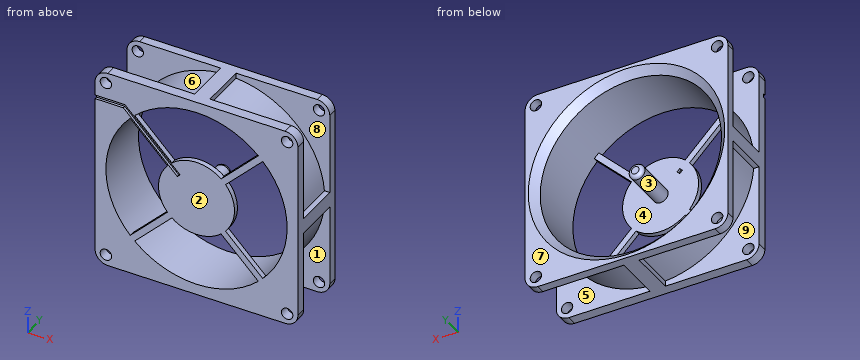
```python
from build123d import *

# Parameters (mm, degrees)
SKETCH1_W            = 80
SKETCH1_H            = 80
BOSS_EXTRUDE1_DEPTH  = 25.5
SKETCH2_R            = 35.75
CUT_EXTRUDE2_DEPTH   = 28
BOSS_EXTRUDE2_DEPTH  = 2
CIRPATTERN2_COUNT    = 4
SKETCH5_R            = 15
BOSS_EXTRUDE3_DEPTH  = 2
SKETCH6_R            = 3
BOSS_EXTRUDE4_DEPTH  = 17.5
FILLET1_R            = 1.5
SKETCH7_R            = 70
SKETCH7_R_2          = 38
CUT_EXTRUDE4_DEPTH   = 18
FILLET2_R            = 5
BOSS_EXTRUDE5_DEPTH  = 20
CIRPATTERN3_COUNT    = 4
SKETCH9_R            = 2.25
CUT_EXTRUDE5_DEPTH   = 37
LPATTERN1_COUNT      = 2
LPATTERN1_PITCH      = 71.5
LPATTERN1_COUNT_DIR2 = 2
LPATTERN1_PITCH_DIR2 = 71.5
CHAMFER2_SIZE        = 3
CUT_EXTRUDE6_DEPTH   = 1
CUT_EXTRUDE7_DEPTH   = 7


with BuildPart() as part:
    # Sketch1 → Boss-Extrude1 (new body)
    with BuildSketch(Plane(origin=(0, 0, 0), x_dir=(1, 0, 0), z_dir=(0, 1, 0))):
        Rectangle(SKETCH1_W, SKETCH1_H)
    extrude(amount=BOSS_EXTRUDE1_DEPTH)

    # Sketch2 → Cut-Extrude2 (cut)
    with BuildSketch(Plane(origin=(0, 25.5, 0), x_dir=(1, 0, 0), z_dir=(0, 1, 0))):
        Circle(SKETCH2_R)
    extrude(amount=-CUT_EXTRUDE2_DEPTH, mode=Mode.SUBTRACT)

    # Sketch4 → Boss-Extrude2 (add)
    with BuildSketch(Plane.XZ):
        with BuildLine():
            Line((-1.75, 0), (0, 1.785533906))
            Line((0, 1.785533906), (-24.370530875, 26.156064781))
            ThreePointArc((-24.370530875, 26.156064781), (-25.270176953, 25.287954776), (-26.138919431, 24.388919431))
            Line((-26.138919431, 24.388919431), (-1.75, 0))
        make_face()
    boss_extrude2 = extrude(amount=-BOSS_EXTRUDE2_DEPTH)

    # CirPattern2: Boss-Extrude2 ×4 about axis
    cirpattern2_axis = Axis((0, 0, 0), (0, 1, 0))
    for i in range(1, CIRPATTERN2_COUNT):
        add(boss_extrude2.rotate(cirpattern2_axis, i * 360 / CIRPATTERN2_COUNT))

    # Sketch5 → Boss-Extrude3 (add)
    with BuildSketch(Plane.XZ):
        Circle(SKETCH5_R)
    extrude(amount=-BOSS_EXTRUDE3_DEPTH)

    # Sketch6 → Boss-Extrude4 (add)
    with BuildSketch(Plane(origin=(0, 2, 0), x_dir=(1, 0, 0), z_dir=(0, 1, 0))):
        Circle(SKETCH6_R)
    extrude(amount=BOSS_EXTRUDE4_DEPTH)

    # Fillet1
    fillet1_edges = [part.edges().sort_by_distance(p)[0] for p in [
        (-3, 19.5, 0),
    ]]
    fillet(fillet1_edges, radius=FILLET1_R)

    # Sketch7 → Cut-Extrude4 (cut)
    with BuildSketch(Plane.XZ.offset(-4)):
        Circle(SKETCH7_R)
        Circle(SKETCH7_R_2, mode=Mode.SUBTRACT)
    extrude(amount=-CUT_EXTRUDE4_DEPTH, mode=Mode.SUBTRACT)

    # Fillet2
    fillet2_edges = [part.edges().sort_by_distance(p)[0] for p in [
        (-40, 2, -40),
        (40, 2, -40),
        (40, 2, 40),
        (-40, 2, 40),
        (-40, 23.75, -40),
        (40, 23.75, -40),
        (40, 23.75, 40),
        (-40, 23.75, 40),
    ]]
    fillet(fillet2_edges, radius=FILLET2_R)

    # Sketch8 → Boss-Extrude5 (add)
    with BuildSketch(Plane.XZ.offset(-4)):
        with BuildLine():
            Line((-3, 40), (3, 40))
            Line((3, 40), (3, 35.623903492))
            ThreePointArc((3, 35.623903492), (0, 35.75), (-3, 35.623903492))
            Line((-3, 35.623903492), (-3, 40))
        make_face()
    boss_extrude5 = extrude(amount=-BOSS_EXTRUDE5_DEPTH)

    # CirPattern3: Boss-Extrude5 ×4 about axis
    cirpattern3_axis = Axis((0, 0, 0), (0, 1, 0))
    for i in range(1, CIRPATTERN3_COUNT):
        add(boss_extrude5.rotate(cirpattern3_axis, i * 360 / CIRPATTERN3_COUNT))

    # Sketch9 → Cut-Extrude5 (cut)
    with BuildSketch(Plane(origin=(0, 25.5, 0), x_dir=(-1, 0, 0), z_dir=(0, 1, 0))):
        with Locations((35.75, -35.75)):
            Circle(SKETCH9_R)
    cut_extrude5 = extrude(amount=-CUT_EXTRUDE5_DEPTH, mode=Mode.SUBTRACT)

    # LPattern1: Cut-Extrude5 2 × 2
    with Locations(*[(i * LPATTERN1_PITCH, 0, j * LPATTERN1_PITCH_DIR2) for i in range(LPATTERN1_COUNT) for j in range(LPATTERN1_COUNT_DIR2) if (i, j) != (0, 0)]):
        add(cut_extrude5, mode=Mode.SUBTRACT)

    # Chamfer2
    chamfer2_edges = [part.edges().sort_by_distance(p)[0] for p in [
        (-35.75, 25.5, 0),
    ]]
    chamfer(chamfer2_edges, length=CHAMFER2_SIZE)

    # Sketch11 → Cut-Extrude6 (cut)
    with BuildSketch(Plane.XZ):
        Polygon((-28.863216429, 27.820323211), (-7.554875149, 6.51198193), (-6.494214977, 7.572642102), (-28.241896086, 29.320323211), (-40, 29.320323211), (-40, 27.820323211), align=None)
    extrude(amount=-CUT_EXTRUDE6_DEPTH, mode=Mode.SUBTRACT)

    # Sketch12 → Cut-Extrude7 (cut)
    with BuildSketch(Plane.XZ.offset(-1)):
        Polygon((-6.494214977, 7.572642102), (-7.554875149, 8.633302273), (-8.61553532, 7.572642102), (-7.554875149, 6.51198193), align=None)
    extrude(amount=-CUT_EXTRUDE7_DEPTH, mode=Mode.SUBTRACT)


solid = part.part
```
CAD build for the part. Positions are in the model's coordinates, mm. Face numbers are marked on the shaded views. A direction names the side the tool comes from. Coordinates: 2 decimals unless noted, no trailing zeros. Write each loop counter-clockwise with the first axis right and the second up, starting at its lowest first coordinate (ties: lowest second). Pieces come first, ordered by that corner, then holes. Notation, with made-up numbers: (12, 85.25) -> (68, 85.25) arc R16 ccw to (68, 105.25) -> close; hole circle Ø3 at (75.25, 42). An arc over 180 degrees is marked (long way). Return JSON: item names as keys, results as strings. Group by question number.
Q1. Cut at A-A, the plane y = 10.75. Give the cut face in (x, z), then the cut area to 3 significant figures.
Q2. Flat gauge pins, fed straight in: pin 1 (8 mm diameter, centred on x = -6, y = 15, fed in from +Z); pin 2 (0.6 mm diameter, centred on y = 15, z = 39, fed in from -X); pin 3 (11 mm diameter, centred on x = 16, z = 16, fed in from +Y); pin 4 (1.5 mm diameter, centred on y = 17.5, z = 14, fed in from +X). Where does each tip first touch, or does it go through?
Q3. Drill centre lines: line 1 (X direction, y = 8.25, z = 0); line 2 (Y direction, x = 27, z = 34.5); line 3 (X direction, y = 19, z = -0.5). Where is each one in solid material? Low to high.
Q4. Pull direction Y, two halves, no side cores. Call the marked faces 1, 2, 3 and 4: released by +Y, released by -Y, zero draft, split by the parting line, or undercut.
Q5. Which spindle directions (+Z, -Z, +X, -X, +Y, -Y) get a long thin tool onto all of the face, cutting with end or side? Do the marked faces 5, 6, 7, 8 and 9. Say none if no direction does.
Q6. Cut at B-B, the plane z = 0. State how many separate pieces and enclosed holes the cut face has, then the cut area to 3 significant figures.
Returned:
{
 "1": {"outline": "(-40, -3) -> (-37.88, -3) arc R38 ccw to (-3, -37.88) -> (-3, -40) -> (3, -40) -> (3, -37.88) arc R38 ccw to (37.88, -3) -> (40, -3) -> (40, 3) -> (37.88, 3) arc R38 ccw to (3, 37.88) -> (3, 40) -> (-3, 40) -> (-3, 37.88) arc R38 ccw to (-37.88, 3) -> (-40, 3) -> close; circle Ø6 at (0, 0); hole circle Ø71.5 at (0, 0)", "area": "599 mm2"},
 "2": {"pin 1": "stops at z = 40", "pin 2": "stops at x = -3", "pin 3": "stops at y = 2", "pin 4": "stops at x = 35.62"},
 "3": {"line 1": "x = -40 to -35.75, -3 to 3, 35.75 to 40", "line 2": "y = 0 to 4, 22 to 25.5", "line 3": "x = -40 to -35.75, -2.57 to 2.57, 35.75 to 40"},
 "4": {"face 1": "undercut", "face 2": "released by -Y", "face 3": "zero draft", "face 4": "released by +Y"},
 "5": {"face 5": "-Z, +X", "face 6": "+Z, -X", "face 7": "+Z, -Z, +X, -X, +Y", "face 8": "+Z, +X", "face 9": "-Z, -X"},
 "6": {"separate pieces": "3", "enclosed holes": "0", "area": "372 mm2"}
}
